Geometry check sheet. Reference: drawing and pictorial views, mm from the part's lowest x, y, z. A direction names the side the tool comes from. Round coordinates to 2 decimals unless told otherwise and drop trailing zeros. Order: outer loops, then holes, each group sorted by start corner. A loop starts at its lowest first (then second) coordinate and runs counter-clockwise, first axis right, second up.
(1) Tool access check on the marked faces 1, 2, 3 and 4. Record the directions out of +Z, -Z, +X, -X, +Y, -Y that give a thin tool (end or side, any length) a straight path to the whole face; none if there is none.
(2) Sectioned sample at A-A, the plane z = 33. Enter the section's corners in (x, y), and give its area (3 significant figures).
(3) Sectioned sample at D-D, the plane y = 25.5. Enter the section's corners in (x, z), and give its area (3 significant figures).
(4) Sectioned sample at B-B, the plane x = 6. Enter the section's corners in (y, z).
(5) Thickness scan on probe 1 along Y at (x, z) = (45.5, 28.5); probe 2 along Z at (x, y) = (11.5, 11.5); probe 3 along X at (y, z) = (56, 15). Record the ranges inside material, lowest first.
(6) Depth check by flat-ended pin: pin 1 (3 mm diameter, centred on x = 11.5, z = 15.5, fed in from +Y); pin 2 (11 mm diameter, centred on x = 25.5, z = 11, fed in from +Y); pin 3 (2 mm diameter, centred on x = 29, y = 30.5, fed in from +Z). Enter the tip coordinate at first touch or a pass-through.
(7) Sectioned sample at C-C, the plane z = 5. Enter the section's corners in (x, y), and give its area (3 significant figures).
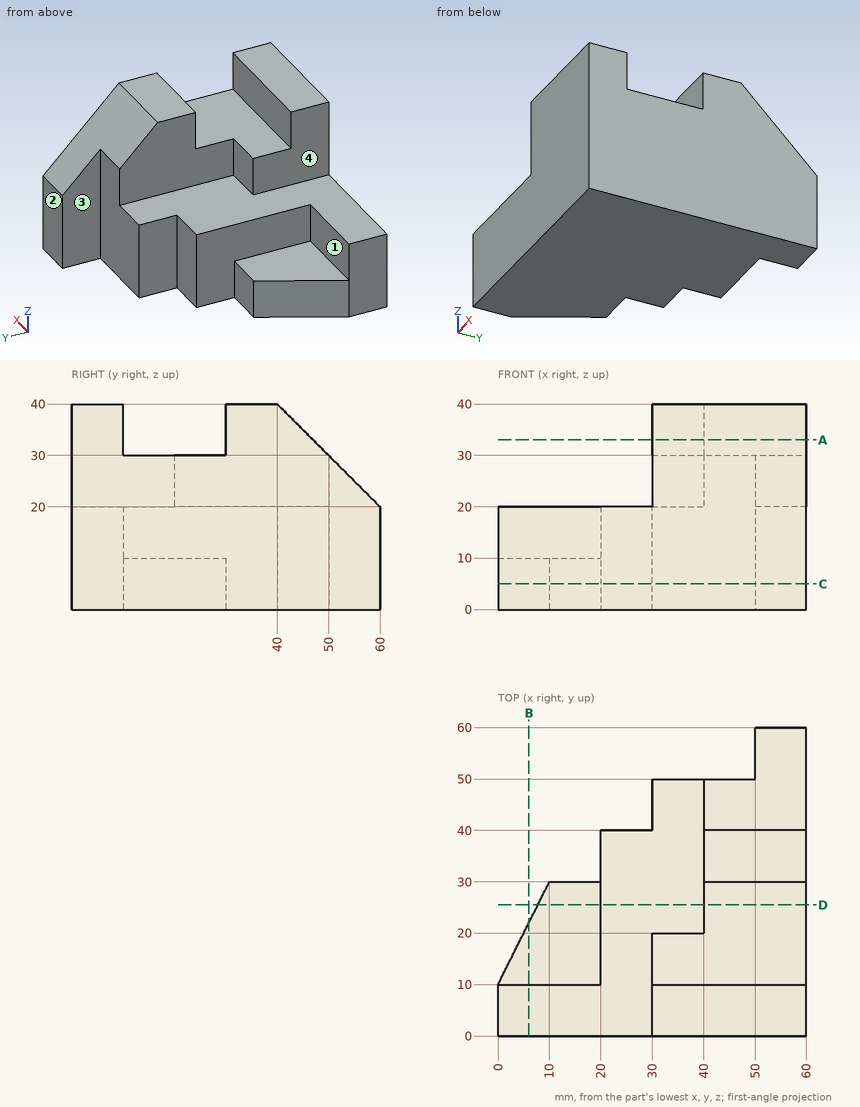
Derived:
1. face 1: +Z, -X, +Y
1. face 2: +Z, -Z, +X, -X, +Y
1. face 3: +Z, -Z, -X, +Y
1. face 4: +Z, -X, +Y, -Y
2. outline: (30, 0) - (60, 0) - (60, 10) - (30, 10) - close; (40, 30) - (60, 30) - (60, 47) - (40, 47) - close
2. area: 640 mm2
3. outline: (7.75, 0) - (60, 0) - (60, 30) - (40, 30) - (40, 20) - (20, 20) - (20, 10) - (7.75, 10) - close
3. area: 1,120 mm2
4. outline: (0, 0) - (22, 0) - (22, 10) - (10, 10) - (10, 20) - (0, 20) - close
5. probe 1: y = 0 to 50
5. probe 2: z = 0 to 10
5. probe 3: x = 50 to 60
6. pin 1: stops at y = 10
6. pin 2: stops at y = 50
6. pin 3: stops at z = 20
7. outline: (0, 0) - (60, 0) - (60, 60) - (50, 60) - (50, 50) - (30, 50) - (30, 40) - (20, 40) - (20, 30) - (10, 30) - (0, 10) - close
7. area: 2,500 mm2
